from build123d import *

# Parameters (mm, degrees)
SKETCH1_R          = 24
BASE_FLANGE1_DEPTH = 2
SKETCH6_R          = 2.1
SKETCH6_W          = 3.18
SKETCH6_H          = 3.18
CUT_EXTRUDE1_DEPTH = 10
SKETCH8_R          = 24
SKETCH8_R_2        = 22.5
CUT_EXTRUDE3_DEPTH = 10


# Sheet-metal steps are written as plain solids
with BuildPart() as part:
    # Sketch1 → Base-Flange1 (new body)
    with BuildSketch(Plane.XY):
        Circle(SKETCH1_R)
    extrude(amount=-BASE_FLANGE1_DEPTH)

    # Sketch6 → Cut-Extrude1 (cut)
    with BuildSketch(Plane.XY):
        with Locations((-12.7, 12.7)):
            Circle(SKETCH6_R)
        with Locations((12.7, 12.7)):
            Circle(SKETCH6_R)
        with Locations((12.7, -12.7)):
            Circle(SKETCH6_R)
        with Locations((-12.7, -12.7)):
            Circle(SKETCH6_R)
        Rectangle(SKETCH6_W, SKETCH6_H)
    extrude(amount=-CUT_EXTRUDE1_DEPTH, mode=Mode.SUBTRACT)

    # Sketch8 → Cut-Extrude3 (cut)
    with BuildSketch(Plane.XY):
        Circle(SKETCH8_R)
        Circle(SKETCH8_R_2, mode=Mode.SUBTRACT)
    extrude(amount=-CUT_EXTRUDE3_DEPTH, mode=Mode.SUBTRACT)


solid = part.part
For this review, take the finished solid that the model builds, in its own axes (mm). A direction names the side the tool comes from. Give positions to 0.01 mm unless a question says otherwise; leave off trailing zeros. Loops run counter-clockwise (first coordinate to the right, second up) from the corner with the lowest first, then second, coordinate; pieces in that order, holes last. Notation, with made-up numbers: M 71,-2.75 L 119,-2.75 A7 cw 119,10.25 Z; hole C 59.25,36 d11. An arc over 180 degrees is marked long. Put each result on its own line as item: value. Start each with the question number.
(1) Machinability: for faces 5 (the flat face through (-1.59, 0, -1)), 6 (the flat face through (5, 0, -2)), which of the approach directions +Z, -Z, +X, -X, +Y, -Y give a long, thin tool a straight path to every point of the face, cutting with its end or side? Answer none if there is none.
(2) Add section A-A, the plane y = 0. Write out the cut boundary in (x, z).
(3) For pin 1 (2.5 mm diameter, centred on x = 12.7, y = -12.7, fed in from -Z), flat-tipped, find the tip position at first contact; note if it passes through.
(4) Wall thickness on L1, parallel to Y at x = 12.7, z = -0.5; L2, parallel to X at y = -11.5, z = -0.7; L3, parallel to Y at x = -0.5, z = -0.8: over which ranges is each line inside the solid? List them lowest first.
(5) The part is to be moulded in two halves that separate along X. For faces 1 (the flat face through (0, 1.59, -1)), 2 (the cylindrical face through (10.382, -19.961, -0.986)), 3 (the flat face through (5, 0, 0)), 4 (the cylindrical face through (12.24, -14.75, -0.99)), say which applies: +X half, -X half, draft (parallel to the pull), parting line (faces both ways), or undercut.
(6) Add section D-D, the plane x = -12.7. Write out the cut boundary in (y, z), then the cut area to 3 significant figures.
(7) Add section C-C, the plane z = -1.3. Write out the cut boundary in (x, y), then the cut area to 3 significant figures.
Result:
1. face 5: +Z, -Z
1. face 6: -Z, +X, -X, +Y, -Y
2. outline: M -22.5,-2 L -1.59,-2 L -1.59,0 L -22.5,0 Z; M 1.59,-2 L 22.5,-2 L 22.5,0 L 1.59,0 Z
3. pin 1: passes through
4. L1: y = -18.57 to -14.8, -10.6 to 10.6, 14.8 to 18.57
4. L2: x = -19.34 to -14.42, -10.98 to 10.98, 14.42 to 19.34
4. L3: y = -22.49 to -1.59, 1.59 to 22.49
5. face 1: undercut
5. face 2: parting line
5. face 3: draft
5. face 4: undercut
6. outline: M -18.57,-2 L -14.8,-2 L -14.8,0 L -18.57,0 Z; M -10.6,-2 L 10.6,-2 L 10.6,0 L -10.6,0 Z; M 14.8,-2 L 18.57,-2 L 18.57,0 L 14.8,0 Z
6. area: 57.5 mm^2
7. outline: C 0,0 d45; hole C -12.7,-12.7 d4.2; hole C -12.7,12.7 d4.2; hole M -1.59,-1.59 L 1.59,-1.59 L 1.59,1.59 L -1.59,1.59 Z; hole C 12.7,-12.7 d4.2; hole C 12.7,12.7 d4.2
7. area: 1,520 mm^2
